from build123d import *

# Parameters (mm, degrees)
SKETCH1_W           = 11.699975178
SKETCH1_H           = 11.699996949
SKETCH1_W_2         = 11.699990436
SKETCH1_H_2         = 11.699981689
SKETCH1_W_3         = 11.699990437
SKETCH1_H_3         = 11.699975177
SKETCH1_W_4         = 11.699981689
SKETCH1_H_4         = 11.699990436
BOSS_EXTRUDE1_DEPTH = 1907.794


with BuildPart() as part:
    # Sketch1 → Boss-Extrude1 (new body)
    with BuildSketch(Plane.XY):
        Polygon((-4.249491247, 17.999291576), (-4.249490956, 22.199304807), (-4.249490956, 22.499297883), (-22.499484399, 22.499298105), (-22.499484948, -22.500701346), (22.500514502, -22.500701895), (22.500515052, 22.499297556), (4.250509108, 22.499297779), (4.250509108, 22.199304487), (4.250508817, 17.999291575), (6.800527063, 17.999291575), (6.800526453, 9.199302988), (4.800526064, 7.199302969), (-4.799479817, 7.199303635), (-6.799479854, 9.199304042), (-6.799479244, 17.999291576), align=None)
        with Locations((-14.649542346, -14.650709384)):
            Rectangle(SKETCH1_W, SKETCH1_H, mode=Mode.SUBTRACT)
        with BuildLine():
            Line((-22.199510799, -4.250714391), (-22.199510799, -3.950696126))
            Line((-22.199510799, -3.950696126), (-21.731790056, -3.48300681))
            ThreePointArc((-21.731790056, -3.48300681), (-21.189814855, -2.671927844), (-20.999497617, -1.71518046))
            Line((-20.999497617, -1.71518046), (-20.999497617, 1.713721031))
            ThreePointArc((-20.999497617, 1.713721031), (-21.189799286, 2.670430863), (-21.731732544, 3.481489907))
            Line((-21.731732544, 3.481489907), (-22.199510888, 3.949267256))
            Line((-22.199510888, 3.949267256), (-22.199510888, 4.249285566))
            Line((-22.199510888, 4.249285566), (-17.999497356, 4.249285704))
            Line((-17.999497356, 4.249285704), (-17.999497356, 6.79927354))
            Line((-17.999497356, 6.79927354), (-9.199509947, 6.799273828))
            Line((-9.199509947, 6.799273828), (-7.199509956, 4.799274012))
            Line((-7.199509956, 4.799274012), (-7.199509641, -4.800732197))
            Line((-7.199509641, -4.800732197), (-9.199509449, -6.800732179))
            Line((-9.199509449, -6.800732179), (-17.99949762, -6.800732468))
            Line((-17.99949762, -6.800732468), (-17.99949762, -4.250714253))
            Line((-17.99949762, -4.250714253), (-22.199510799, -4.250714391))
        make_face(mode=Mode.SUBTRACT)
        with BuildLine():
            Line((-4.24949208, -18.000719999), (-6.799479919, -18.000719999))
            Line((-6.799479919, -18.000719999), (-6.799480207, -9.200732353))
            Line((-6.799480207, -9.200732353), (-4.799480391, -7.200732362))
            Line((-4.799480391, -7.200732362), (4.800525817, -7.200732047))
            Line((4.800525817, -7.200732047), (6.8005258, -9.200731855))
            Line((6.8005258, -9.200731855), (6.800526088, -18.000720263))
            Line((6.800526088, -18.000720263), (4.250507877, -18.000720263))
            Line((4.250507877, -18.000720263), (4.250508015, -22.200733153))
            Line((4.250508015, -22.200733153), (3.950489751, -22.200733153))
            Line((3.950489751, -22.200733153), (3.482800434, -21.73301241))
            ThreePointArc((3.482800434, -21.73301241), (2.671721468, -21.191037209), (1.714974084, -21.000719971))
            Line((1.714974084, -21.000719971), (-1.713927407, -21.000719971))
            ThreePointArc((-1.713927407, -21.000719971), (-2.670637239, -21.19102164), (-3.481696283, -21.732954898))
            Line((-3.481696283, -21.732954898), (-3.949473632, -22.200733242))
            Line((-3.949473632, -22.200733242), (-4.249491942, -22.200733242))
            Line((-4.249491942, -22.200733242), (-4.24949208, -18.000719999))
        make_face(mode=Mode.SUBTRACT)
        with Locations((14.65050626, -14.650767962)):
            Rectangle(SKETCH1_W_2, SKETCH1_H_2, mode=Mode.SUBTRACT)
        with BuildLine():
            Line((-3.181457266, -4.596908447), (-4.595670829, -3.182694885))
            Line((-4.595670829, -3.182694885), (-3.26221457, -1.849238626))
            ThreePointArc((-3.26221457, -1.849238626), (-3.749476751, -0.00071437), (-3.26221457, 1.847809887))
            Line((-3.26221457, 1.847809887), (-4.595670829, 3.181266146))
            Line((-4.595670829, 3.181266146), (-3.181457266, 4.595479708))
            Line((-3.181457266, 4.595479708), (-1.848001007, 3.262023449))
            ThreePointArc((-1.848001007, 3.262023449), (0.000523249, 3.74928563), (1.849047505, 3.262023449))
            Line((1.849047505, 3.262023449), (3.182503764, 4.595479708))
            Line((3.182503764, 4.595479708), (4.596717327, 3.181266146))
            Line((4.596717327, 3.181266146), (3.263261068, 1.847809887))
            ThreePointArc((3.263261068, 1.847809887), (3.750523249, -0.00071437), (3.263261068, -1.849238626))
            Line((3.263261068, -1.849238626), (4.596717327, -3.182694885))
            Line((4.596717327, -3.182694885), (3.182503764, -4.596908447))
            Line((3.182503764, -4.596908447), (1.849047505, -3.263452188))
            ThreePointArc((1.849047505, -3.263452188), (0.000523249, -3.75071437), (-1.848001007, -3.263452188))
            Line((-1.848001007, -3.263452188), (-3.181457266, -4.596908447))
        make_face(mode=Mode.SUBTRACT)
        with Locations((-14.64949028, 14.649335967)):
            Rectangle(SKETCH1_W_3, SKETCH1_H_3, mode=Mode.SUBTRACT)
        with BuildLine():
            Line((9.200519462, -6.800702567), (7.200519471, -4.800702751))
            Line((7.200519471, -4.800702751), (7.200519156, 4.799303458))
            Line((7.200519156, 4.799303458), (9.200518964, 6.79930344))
            Line((9.200518964, 6.79930344), (18.000507424, 6.799303729))
            Line((18.000507424, 6.799303729), (18.000507424, 4.249285514))
            Line((18.000507424, 4.249285514), (22.200520261, 4.249285652))
            Line((22.200520261, 4.249285652), (22.200520261, 3.949267391))
            Line((22.200520261, 3.949267391), (21.732799519, 3.481578075))
            ThreePointArc((21.732799519, 3.481578075), (21.190824318, 2.670499108), (21.000507079, 1.713751724))
            Line((21.000507079, 1.713751724), (21.000507079, -1.715149766))
            ThreePointArc((21.000507079, -1.715149766), (21.190808749, -2.671859599), (21.732742007, -3.482918643))
            Line((21.732742007, -3.482918643), (22.200520351, -3.950695992))
            Line((22.200520351, -3.950695992), (22.200520351, -4.250714302))
            Line((22.200520351, -4.250714302), (18.000507108, -4.25071444))
            Line((18.000507108, -4.25071444), (18.000507108, -6.800702279))
            Line((18.000507108, -6.800702279), (9.200519462, -6.800702567))
        make_face(mode=Mode.SUBTRACT)
        with Locations((14.650561583, 14.6492839)):
            Rectangle(SKETCH1_W_4, SKETCH1_H_4, mode=Mode.SUBTRACT)
    extrude(amount=BOSS_EXTRUDE1_DEPTH)


solid = part.part
Check sheet for the modelled part. Datum: model origin and axes. Units: mm. Round coordinates to 2 decimals unless told otherwise and drop trailing zeros.
1. Sectioned sample at A-A on z = 1580. Give the number of separate pieces and of enclosed holes in the cut face, and give its area (3 significant figures).
2. Scan lines: probe 1 along Y at (x, z) = (6.5, 516.5); probe 2 along X at (y, z) = (-17.5, 1706). Record each from-to range of solid material in increasing order.
3. Gauge pin test, flat end, axial feed: pin 1 Ø4 at (x, y) = (-13.5, 12.5) entering from +Z. Record the tip position at first contact, or that the pin passes through.
Recorded:
1. separate pieces: 1
1. enclosed holes: 8
1. area: 725 mm2
2. probe 1: y = -22.5 to -18, -8.9 to 8.9, 18 to 22.5
2. probe 2: x = -22.5 to -20.5, -8.8 to -6.8, 6.8 to 8.8, 20.5 to 22.5
3. pin 1: passes through
